```python
from build123d import *

# Parameters (mm, degrees)
SKETCH1_W           = 49
SKETCH1_H           = 40
SKETCH1_R           = 1.5
BOSS_EXTRUDE1_DEPTH = 6
CUT_EXTRUDE1_DEPTH  = 0.05


with BuildPart() as part:
    # Sketch1 → Boss-Extrude1 (new body)
    with BuildSketch(Plane(origin=(0, 0, 0), x_dir=(1, 0, 0), z_dir=(0, 1, 0))):
        Rectangle(SKETCH1_W, SKETCH1_H)
        with Locations((-15.25, 15.25)):
            Circle(SKETCH1_R, mode=Mode.SUBTRACT)
        with Locations((15.25, 15.25)):
            Circle(SKETCH1_R, mode=Mode.SUBTRACT)
        with Locations((15.25, -15.25)):
            Circle(SKETCH1_R, mode=Mode.SUBTRACT)
        with Locations((-15.25, -15.25)):
            Circle(SKETCH1_R, mode=Mode.SUBTRACT)
    extrude(amount=BOSS_EXTRUDE1_DEPTH)

    # Sketch2 → Cut-Extrude1 (cut)
    with BuildSketch(Plane(origin=(0, 6, 0), x_dir=(1, 0, 0), z_dir=(0, 1, 0))):
        Polygon((0.269230769, 0), (0.731270032, 3.5), (0.776141827, 3.5), (2.221153846, 0.628205128), (3.661959135, 3.5), (3.706830929, 3.5), (4.173076923, 0), (3.858974359, 0), (3.522435897, 2.516326122), (2.259715545, 0), (2.188201122, 0), (0.919871795, 2.524038462), (0.585436699, 0), align=None)
        Polygon((6.326923077, 3.5), (7.942307692, 0), (7.600861378, 0), (7.083433494, 1.121794872), (5.496794872, 1.121794872), (4.965344551, 0), (4.621794872, 0), (6.282051282, 3.5), align=None)
        Polygon((6.300981571, 2.817107372), (5.66786859, 1.480769231), (6.91796875, 1.480769231), align=None, mode=Mode.SUBTRACT)
        Polygon((8.166666667, 3.141025641), (8.166666667, 3.5), (10.006410256, 3.5), (10.006410256, 3.141025641), (9.243589744, 3.141025641), (9.243589744, 0), (8.929487179, 0), (8.929487179, 3.141025641), align=None)
        Polygon((10.544871795, 3.5), (12.519230769, 3.5), (12.519230769, 3.141025641), (10.858974359, 3.141025641), (10.858974359, 2.064102564), (12.519230769, 2.064102564), (12.519230769, 1.705128205), (10.858974359, 1.705128205), (10.858974359, 0.358974359), (12.519230769, 0.358974359), (12.519230769, 0), (10.544871795, 0), align=None)
        Polygon((13.147435897, 3.5), (13.461538462, 3.5), (13.461538462, 2.167167468), (14.920572917, 3.5), (15.368589744, 3.5), (13.648737981, 1.929487179), (15.503205128, 0), (15.083934295, 0), (13.461538462, 1.689002404), (13.461538462, 0), (13.147435897, 0), align=None)
    extrude(amount=-CUT_EXTRUDE1_DEPTH, mode=Mode.SUBTRACT)


solid = part.part
```
Geometry check sheet. Reference: the model listing, model coordinates, mm. Coordinates: 2 decimals unless noted, no trailing zeros. Order: outer loops, then holes, each group sorted by start corner. A loop starts at its lowest first (then second) coordinate and runs counter-clockwise, first axis right, second up.
Q1. Thickness scan on probe 1 along Z at (x, y) = (-15.25, 2.05); probe 2 along X at (y, z) = (2.5, 15.25); probe 3 along X at (y, z) = (4.55, 14). Record the ranges inside material, lowest first.
Reply:
probe 1: z = -20 to -16.75, -13.75 to 13.75, 16.75 to 20
probe 2: x = -24.5 to -16.75, -13.75 to 13.75, 16.75 to 24.5
probe 3: x = -24.5 to -16.08, -14.42 to 14.42, 16.08 to 24.5
Q2. Draft check along X on faces 1 (the face through (-16.75, 2.96, -15.32)), 2 (the face through (13.75, 2.96, -15.32)), 3 (the face through (-24.5, 3, 0)), 4 (the face through (24.5, 3, 0)). Enter one of: released by +X, released by -X, zero draft, split by the parting line, or undercut.
Reply:
face 1: undercut
face 2: undercut
face 3: released by -X
face 4: released by +X
Q3. Sectioned sample at A-A on z = -15.25. Record the cut outline in (x, y), and give its area (3 significant figures).
Reply:
outline: (-24.5, 0) - (-16.75, 0) - (-16.75, 6) - (-24.5, 6) - close; (-13.75, 0) - (13.75, 0) - (13.75, 6) - (-13.75, 6) - close; (16.75, 0) - (24.5, 0) - (24.5, 6) - (16.75, 6) - close
area: 258 mm2
